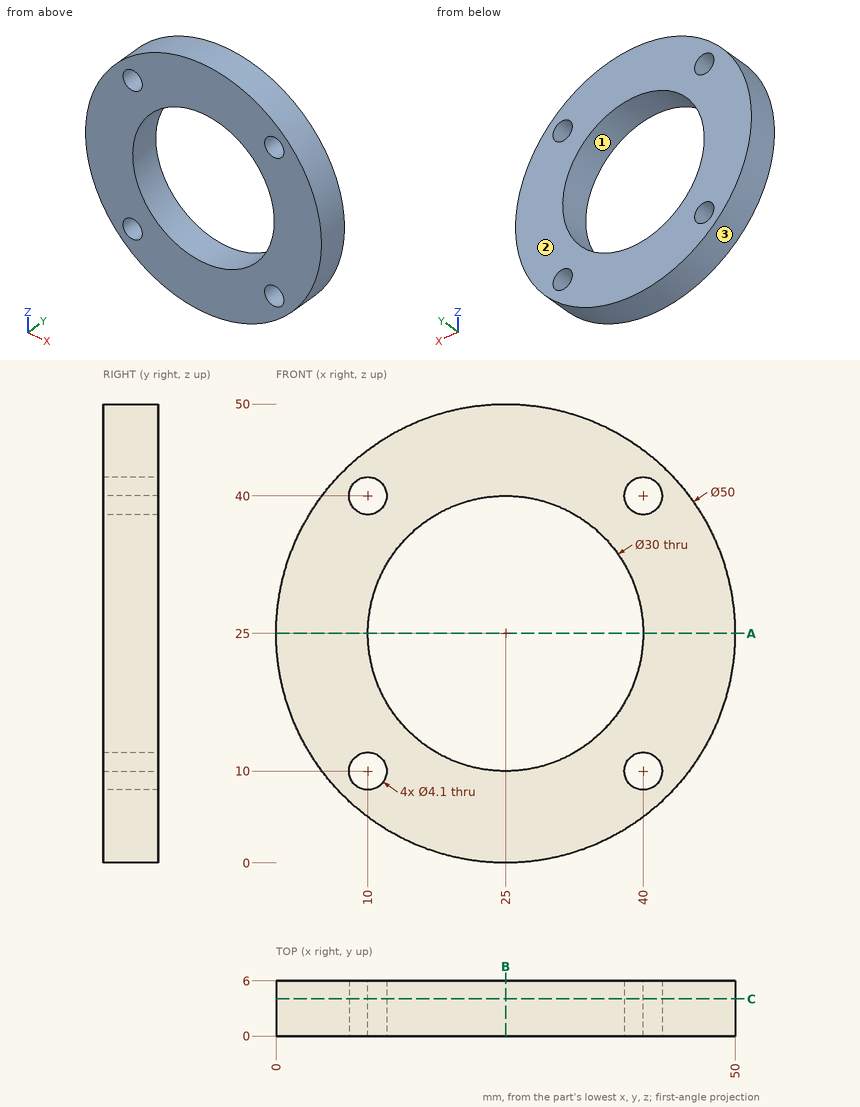
The drawing under review shows one solid part. Ordinate dimensions are in mm from its lowest x, y, z. Coordinates: 2 decimals unless noted, no trailing zeros. Order: outer loops, then holes, each group sorted by start corner. A loop starts at its lowest first (then second) coordinate and runs counter-clockwise, first axis right, second up. Notation, with made-up numbers: (7.25, 50.5) -> (23.25, 50.5) arc R37 ccw to (23.25, 87.5) -> close; hole circle Ø6 at (17, 20). An arc over 180 degrees is marked (long way). Answer in a Markdown table with one row per item.
(1) Consider section C-C (y = 4.05). Write out the cut boundary in (x, z).
Answers:
| item | result |
|---|---|
| outline | circle Ø50 at (25, 25); hole circle Ø4.1 at (10, 10); hole circle Ø4.1 at (10, 40); hole circle Ø30 at (25, 25); hole circle Ø4.1 at (40, 10); hole circle Ø4.1 at (40, 40) |
(2) Consider section B-B (x = 25). Write out the cut boundary in (y, z).
Answers:
| item | result |
|---|---|
| outline | (0, 0) -> (6, 0) -> (6, 10) -> (0, 10) -> close; (0, 40) -> (6, 40) -> (6, 50) -> (0, 50) -> close |
(3) Wall thickness on line 1 along X through (y, z) = (2.25, 25); line 2 along Z through (x, y) = (38.5, 3.3); line 3 along Z through (x, y) = (14, 5.55): over which ranges is each line inside the solid? List them lowest first.
Answers:
| item | result |
|---|---|
| line 1 | 0 to 10, 40 to 50 |
| line 2 | 3.96 to 8.6, 11.4 to 18.46, 31.54 to 38.6, 41.4 to 46.04 |
| line 3 | 2.55 to 14.8, 35.2 to 47.45 |
(4) The part is to be moulded in two halves that separate along X. For the marked faces 1, 2 and 3, say which applies: +X half, -X half, draft (parallel to the pull), parting line (faces both ways), or undercut.
Answers:
| item | result |
|---|---|
| face 1 | undercut |
| face 2 | draft |
| face 3 | parting line |
(5) Consider section A-A (z = 25). Write out the cut boundary in (x, y).
Answers:
| item | result |
|---|---|
| outline | (0, 0) -> (10, 0) -> (10, 6) -> (0, 6) -> close; (40, 0) -> (50, 0) -> (50, 6) -> (40, 6) -> close |
(6) Insertion check: pin 1 (3.5 mm diameter, centred on x = 40, z = 10, fed in from -Y) (3 decimals); pin 2 (1 mm diameter, centred on y = 2.5, z = 27.5, fed in from -X). Each pin has a flat end and moves straight along its axis. Give the tip position at first contact, or say it passes through.
Answers:
| item | result |
|---|---|
| pin 1 | through |
| pin 2 | x = 0.08 |
